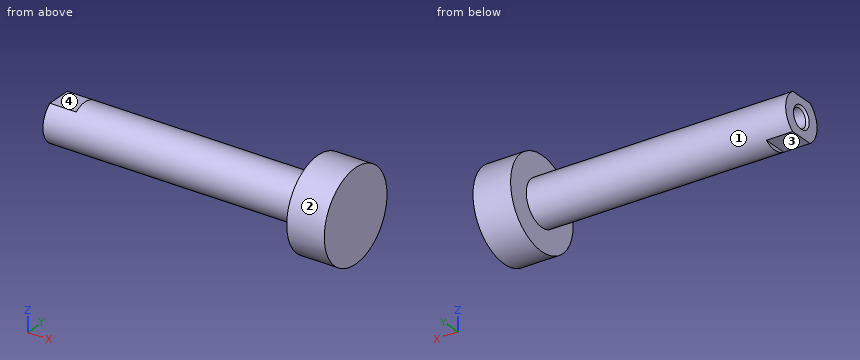
from build123d import *

# Parameters (mm, degrees)
SKETCH1_W                = 5
SKETCH1_H                = 6
SKETCH2_R                = 3
BOSS_EXTRUDE1_DEPTH      = 34.5
CUT_EXTRUDE1_DEPTH       = 3.5
CUT_EXTRUDE2_DEPTH       = 3.5
M2_CLEARANCE_HOLE1_D     = 2.459
M2_CLEARANCE_HOLE1_DEPTH = 6
M2_CLEARANCE_HOLE1_TIP   = 0.709852156
CHAMFER1_SIZE            = 0.2705


with BuildPart() as part:
    # Sketch1 → Revolve1 (revolve)
    with BuildSketch(Plane(origin=(0, 0, 0), x_dir=(-1, 0, 0), z_dir=(0, 0, -1))):
        with Locations((-33.5, 3)):
            Rectangle(SKETCH1_W, SKETCH1_H)
    revolve(axis=Axis((36, 0, 0), (-1, 0, 0)))

    # Sketch2 → Boss-Extrude1 (add)
    with BuildSketch(Plane.ZY.offset(-31)):
        Circle(SKETCH2_R)
    extrude(amount=BOSS_EXTRUDE1_DEPTH)

    # Sketch3 → Cut-Extrude1 (cut)
    with BuildSketch(Plane.ZY.offset(3.5)):
        with BuildLine():
            Line((-2.5, -1.658312395), (-2.5, 1.658312395))
            ThreePointArc((-2.5, 1.658312395), (-3, 0), (-2.5, -1.658312395))
        make_face()
    extrude(amount=-CUT_EXTRUDE1_DEPTH, mode=Mode.SUBTRACT)

    # Sketch4 → Cut-Extrude2 (cut)
    with BuildSketch(Plane.ZY.offset(3.5)):
        with BuildLine():
            Line((2.5, 1.658312395), (2.5, -1.658312395))
            ThreePointArc((2.5, -1.658312395), (3, 0), (2.5, 1.658312395))
        make_face()
    extrude(amount=-CUT_EXTRUDE2_DEPTH, mode=Mode.SUBTRACT)

    # M2 Clearance Hole1
    with Locations(Plane.ZY.offset(3.5)):
        with Locations((0, 0)):
            Hole(M2_CLEARANCE_HOLE1_D / 2, depth=M2_CLEARANCE_HOLE1_DEPTH)
            with Locations((0, 0, -(M2_CLEARANCE_HOLE1_DEPTH + M2_CLEARANCE_HOLE1_TIP / 2))):  # 120° drill point
                Cone(0, M2_CLEARANCE_HOLE1_D / 2, M2_CLEARANCE_HOLE1_TIP, mode=Mode.SUBTRACT)

    # Chamfer1
    chamfer1_edges = [part.edges().sort_by_distance(p)[0] for p in [
        (-3.5, 0, 1.2295),
    ]]
    chamfer(chamfer1_edges, length=CHAMFER1_SIZE)


solid = part.part
Input: part model. Units: mm. Frame: model coordinates. Face numbers are marked on the shaded views. A direction names the side the tool comes from. Give positions to 0.01 mm unless a question says otherwise; leave off trailing zeros. Order: outer loops, then holes, each group sorted by start corner. A loop starts at its lowest first (then second) coordinate and runs counter-clockwise, first axis right, second up. Notation, with made-up numbers: (-6, 47) - (8, 47) arc R25 cw to (8, 61) - close; hole circle Ø11 at (-38, 52). An arc over 180 degrees is marked (long way). Answer as a JSON object with one key per item and string values. Group by question number.
Q1. Cut plane A-A, the plane z = -2. Output: boundary loops of the cut face in (x, y).
Q2. Cut plane B-B, the plane x = 4.5. Output: boundary loops of the cut face in (y, z).
Q3. First-contact query: pin 1 Ø1 at (x, y) = (-2, 0.5) entering from +Z; pin 2 Ø1.5 at (y, z) = (2.5, -3) entering from -X; pin 3 Ø1 at (x, y) = (29.5, -0.5) entering from +Z. Flat tips, straight axial feed; report the tip coordinate or a pass-through.
Q4. Line query: probe 1 along Z at (x, y) = (-1.7, 0); probe 2 along Z at (x, y) = (0.65, 0); probe 3 along X at (y, z) = (-1.5, -5.5). Output: solid intervals per line, ascending.
Q5. Cut plane D-D, the plane z = -4.25. Output: boundary loops of the cut face in (x, y), then the cut area to 3 significant figures.
Q6. Cut plane C-C, the plane z = 5. Output: boundary loops of the cut face in (x, y), then the cut area to 3 significant figures.
Q7. Set-up query: the marked faces 1, 2, 3 and 4. Return all of +Z, -Z, +X, -X, +Y, -Y with unobstructed straight access to the full face (end or side cutting, diameter ignored); none if empty.
Results:
{
 "1": {"outline": "(-3.5, -2.24) - (31, -2.24) - (31, -5.66) - (36, -5.66) - (36, 5.66) - (31, 5.66) - (31, 2.24) - (-3.5, 2.24) - close"},
 "2": {"outline": "circle Ø6 at (0, 0)"},
 "3": {"pin 1": "z = 2.5", "pin 2": "x = 31", "pin 3": "z = 3"},
 "4": {"probe 1": "-2.5 to -1.23, 1.23 to 2.5", "probe 2": "-3 to -1.23, 1.23 to 3", "probe 3": "31 to 36"},
 "5": {"outline": "(31, -4.24) - (36, -4.24) - (36, 4.24) - (31, 4.24) - close", "area": "42.4 mm^2"},
 "6": {"outline": "(31, -3.32) - (36, -3.32) - (36, 3.32) - (31, 3.32) - close", "area": "33.2 mm^2"},
 "7": {"face 1": "-X", "face 2": "+X, -X", "face 3": "-Z, -X, +Y, -Y", "face 4": "+Z, -X, +Y, -Y"}
}
